Source: CAD feature listing. Evaluate the final solid. Frame: model axes, mm. Coordinates: 2 decimals unless noted, no trailing zeros. Loops run counter-clockwise (first coordinate to the right, second up) from the corner with the lowest first, then second, coordinate; pieces in that order, holes last. Notation, with made-up numbers: (79.5, 76) -> (136.5, 76) arc R21 ccw to (136.5, 84) -> close; hole circle Ø2 at (1.25, -33.75). An arc over 180 degrees is marked (long way). Answer as a JSON object with one key per item and string values. Group by question number.
from build123d import *

# Parameters (mm, degrees)
F1_DEPTH = 0.7112
F2_R     = 2.54
F3_DEPTH = 25.4


with BuildPart() as f1:
    # F0 (on Front) → F1 (new body)
    with BuildSketch(Plane.XZ):
        with BuildLine():
            Line((48.109472, 29.950177), (-40.790528, 29.950177))
            ThreePointArc((-40.790528, 29.950177), (-45.280656, 28.090305), (-47.140528, 23.600177))
            Line((-47.140528, 23.600177), (-47.140528, 10.900177))
            ThreePointArc((-47.140528, 10.900177), (-45.280656, 6.410049), (-40.790528, 4.550177))
            Line((-40.790528, 4.550177), (48.109472, 4.550177))
            ThreePointArc((48.109472, 4.550177), (52.599601, 6.410049), (54.459472, 10.900177))
            Line((54.459472, 10.900177), (54.459472, 23.600177))
            ThreePointArc((54.459472, 23.600177), (52.599601, 28.090305), (48.109472, 29.950177))
        make_face()
    extrude(amount=F1_DEPTH)

    # F2 (on face) → F3 (cut)
    with BuildSketch(Plane.XZ.offset(0.7112)):
        with BuildLine():
            ThreePointArc((-36.218528, 17.250177), (-38.758528, 19.790177), (-41.298528, 17.250177))
            ThreePointArc((-41.298528, 17.250177), (-38.758528, 14.710177), (-36.218528, 17.250177))
        make_face()
        with Locations((46.077472, 17.250177)):
            Circle(F2_R)
    extrude(amount=-F3_DEPTH, mode=Mode.SUBTRACT)


solid = f1.part
1. Ray query, L1, parallel to X at y = -0.3, z = 18.75; L2, parallel to Z at x = 48, y = -0.45; L3, parallel to Z at x = -40.5, y = -0.45. Return the intervals inside material, ascending.
2. Mould query, pull axis X, two halves, no side actions, for faces 1 (the face through (3, 0, 17)), 2 (the face through (48.424, -0.361, 16.277)), 3 (the face through (-45.23, -0.35, 28.14)). Classes: pulls with the +X half, pulls with the -X half, needs draft (parallel to the pull), parting line crosses it, or undercut.
3. Section query A-A on y = -0.4. Return loops of the section in (x, z).
4. Section query B-B on z = 7.75. Return loops of the section in (x, y), then the cut area to 3 significant figures.
Solved:
{
 "1": {"L1": "-47.14 to -40.81, -36.71 to 44.03, 48.13 to 54.46", "L2": "4.55 to 15.59, 18.91 to 29.95", "L3": "4.55 to 15.4, 19.1 to 29.95"},
 "2": {"face 1": "needs draft", "face 2": "undercut", "face 3": "pulls with the -X half"},
 "3": {"outline": "(-47.14, 10.9) arc R6.35 ccw to (-40.79, 4.55) -> (48.11, 4.55) arc R6.35 ccw to (54.46, 10.9) -> (54.46, 23.6) arc R6.35 ccw to (48.11, 29.95) -> (-40.79, 29.95) arc R6.35 ccw to (-47.14, 23.6) -> close; hole circle Ø5.08 at (-38.76, 17.25); hole circle Ø5.08 at (46.08, 17.25)"},
 "4": {"outline": "(-46.3, -0.71) -> (53.62, -0.71) -> (53.62, 0) -> (-46.3, 0) -> close", "area": "71.1 mm^2"}
}
